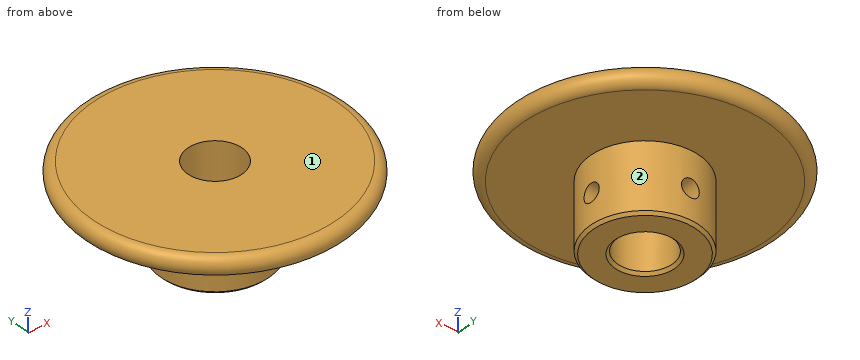
```python
from build123d import *

# Parameters (mm, degrees)
SKETCH_1_R               = 10
EXTRUDE_1_DEPTH          = 12.5
SKETCH_2_R               = 22.5
EXTRUDE_2_DEPTH          = 3.5
SKETCH_4_R               = 5
CUT_EXTRUDE_3_DEPTH      = 36.616007637
SKETCH_5_W               = 1.65
SKETCH_5_H               = 24.25
CHAMFER_2_SIZE           = 0.5
SKETCH_3_R               = 1.75
PATTERN_CIRCULAR_1_COUNT = 2
PATTERN_CIRCULAR_1_ANGLE = 90


with BuildPart() as part:
    # 草图1 → 拉伸1 (new body)
    with BuildSketch(Plane.XY):
        Circle(SKETCH_1_R)
    extrude(amount=EXTRUDE_1_DEPTH)

    # 草图2 → 拉伸2 (add)
    with BuildSketch(Plane.XY.offset(12.5)):
        Circle(SKETCH_2_R)
    extrude(amount=EXTRUDE_2_DEPTH)

    # 草图4 → 拉伸3 (cut, through all)
    with BuildSketch(Plane(origin=(0, 0, 0), x_dir=(-1, 0, 0), z_dir=(0, 0, -1))):
        Circle(SKETCH_4_R)
    extrude(amount=-CUT_EXTRUDE_3_DEPTH, mode=Mode.SUBTRACT)

    # 草图5 → M4 螺纹孔1 (revolve, cut)
    with BuildSketch(Plane(origin=(0, 0, 6), x_dir=(0, 0, -1), z_dir=(1, 0, 0))):
        with Locations((0.825, 12.125)):
            Rectangle(SKETCH_5_W, SKETCH_5_H)
    hole_wizard_m4_1 = revolve(axis=Axis((0, -6.35, 6), (0, 1, 0)), mode=Mode.SUBTRACT)

    # 倒角2
    chamfer_2_edges = [part.edges().sort_by_distance(p)[0] for p in [
        (5, 0, 0),
        (-10, 0, 0),
    ]]
    chamfer(chamfer_2_edges, length=CHAMFER_2_SIZE)

    # 草图3 → 旋转1 (revolve)
    with BuildSketch(Plane(origin=(0, 0, 0), x_dir=(1, 0, 0), z_dir=(0, 1, 0)), mode=Mode.PRIVATE) as revolve_1_sk:
        with Locations((-22.5, -14.25)):
            Circle(SKETCH_3_R)
    revolve(revolve_1_sk.sketch.rotate(Axis((0, 0, 12.5), (0, 0, -1)), 180), axis=Axis((0, 0, 12.5), (0, 0, -1)))

    # 阵列(圆周)1: M4 螺纹孔1 ×2 about axis
    pattern_circular_1_axis = Axis((0, 0, 12.5), (0, 0, -1))
    for i in range(1, PATTERN_CIRCULAR_1_COUNT):
        add(hole_wizard_m4_1.rotate(pattern_circular_1_axis, i * PATTERN_CIRCULAR_1_ANGLE / (PATTERN_CIRCULAR_1_COUNT - 1)), mode=Mode.SUBTRACT)


solid = part.part
```
Here's how the part is built. I have some questions about the finished solid (model axes, mm). Face numbers are marked on the shaded views. A direction names the side the tool comes from. Give positions to 0.01 mm unless a question says otherwise; leave off trailing zeros. Order: outer loops, then holes, each group sorted by start corner. A loop starts at its lowest first (then second) coordinate and runs counter-clockwise, first axis right, second up. Notation, with made-up numbers: (-3.75, 89.5) - (21.25, 89.5) arc R23 ccw to (21.25, 111.5) - close; hole circle Ø5 at (-3.5, 1). An arc over 180 degrees is marked (long way). Answer as a JSON object with one key per item and string values. Group by question number.
Item 1: If we section it at A-A on x = 0: Please give me the cut outline in (y, z).
Item 2: Which directions (+Z, -Z, +X, -X, +Y, -Y) give clear straight access to the entire face, cutting with the end or side of a thin tool? Please do the marked faces 1 and 2.
Item 3: If we section it at D-D on z = 11: Please give me the cut outline in (x, y), and give its area (3 significant figures).
Item 4: If we section it at C-C on z = 5: Please give me the cut outline in (x, y).
Item 5: Please list where these lines run through material, in increasing order: probe 1 along Z at (x, y) = (0, 8.05); probe 2 along Z at (x, y) = (19.5, -8.5); probe 3 along X at (y, z) = (-4.5, 2).
Item 6: For P1, Ø1.5, axis at x = 10.5, z = 12.5, coming from the -Y side; P2, Ø6, axis at x = -5.5, y = 17.5, coming from the -Z side; P3, Ø11.5, axis at x = 0, y = 0, coming from the -Z side; P4, Ø4, axis at x = 16.5, z = 10, coming from the +Y side, each with a flat end and sliding along its axis, tell me the tip position at first contact or that it passes through.
Result set:
{
 "1": {"outline": "(-22.5, 12.5) - (-10, 12.5) - (-10, 0.5) - (-9.5, 0) - (-5.5, 0) - (-5, 0.5) - (-5, 16) - (-22.5, 16) arc R1.75 ccw to start; (5, 0.5) - (5.5, 0) - (9.5, 0) - (10, 0.5) - (10, 4.35) - (5, 4.35) - close; (5, 7.65) - (10, 7.65) - (10, 12.5) - (22.5, 12.5) arc R1.75 ccw to (22.5, 16) - (5, 16) - close"},
 "2": {"face 1": "+Z, +X, -X, +Y, -Y", "face 2": "-Z"},
 "3": {"outline": "circle Ø20 at (0, 0); hole circle Ø10 at (0, 0)", "area": "236 mm²"},
 "4": {"outline": "(-1.31, 4.82) - (-1.31, 9.91) arc R10 ccw (long way) to (9.91, -1.31) - (4.82, -1.31) arc R5 cw (long way) to start; (1.31, 4.82) arc R5 cw to (4.82, 1.31) - (9.91, 1.31) arc R10 ccw to (1.31, 9.91) - close"},
 "5": {"probe 1": "0 to 4.35, 7.65 to 16", "probe 2": "12.5 to 16", "probe 3": "-8.93 to -2.18, 2.18 to 8.93"},
 "6": {"P1": "y = -21.61", "P2": "z = 12.5", "P3": "z = 0", "P4": "through"}
}
